```python
from build123d import *

# Parameters (mm, degrees)
BOARD_DEPTH        = 1.59936
CUT_EXTRUDE2_DEPTH = 2.59936
CUT_EXTRUDE3_DEPTH = 2.59936


with BuildPart() as part:
    # Sketch1 → Board (new body)
    with BuildSketch(Plane.XY):
        with BuildLine():
            Line((10, 12.987), (10, 24.35))
            ThreePointArc((10, 24.35), (10.089703362, 24.915270998), (10.35, 25.425))
            ThreePointArc((10.35, 25.425), (10.610296638, 25.934729002), (10.7, 26.5))
            Line((10.7, 26.5), (10.7, 27.5))
            ThreePointArc((10.7, 27.5), (10.610296638, 28.065270998), (10.35, 28.575))
            ThreePointArc((10.35, 28.575), (10.089703362, 29.084729002), (10, 29.65))
            Line((10, 29.65), (10, 41.1))
            ThreePointArc((10, 41.1), (10.089703362, 41.665270998), (10.35, 42.175))
            ThreePointArc((10.35, 42.175), (10.610296638, 42.684729002), (10.7, 43.25))
            Line((10.7, 43.25), (10.7, 44.25))
            ThreePointArc((10.7, 44.25), (10.610296638, 44.815270998), (10.35, 45.325))
            ThreePointArc((10.35, 45.325), (10.089703362, 45.834729002), (10, 46.4))
            Line((10, 46.4), (10, 57.01299))
            ThreePointArc((10, 57.01299), (10.185195521, 57.290150019), (10.51213, 57.22512))
            ThreePointArc((10.51213, 57.22512), (12.776257609, 57.223732391), (12.77487, 59.48786))
            ThreePointArc((12.77487, 59.48786), (12.709829188, 59.814802566), (12.987, 60))
            Line((12.987, 60), (37.01299, 60))
            ThreePointArc((37.01299, 60), (37.290150019, 59.814804479), (37.22512, 59.48787))
            ThreePointArc((37.22512, 59.48787), (37.223732391, 57.223742391), (39.48786, 57.22513))
            ThreePointArc((39.48786, 57.22513), (39.814807186, 57.290168899), (40, 57.01299))
            Line((40, 57.01299), (40, 12.987))
            ThreePointArc((40, 12.987), (39.814804479, 12.709839981), (39.48787, 12.77487))
            ThreePointArc((39.48787, 12.77487), (37.226515909, 12.773484091), (37.22513, 10.51213))
            ThreePointArc((37.22513, 10.51213), (37.290158106, 10.185190901), (37.01299, 10))
            Line((37.01299, 10), (12.987, 10))
            ThreePointArc((12.987, 10), (12.709839981, 10.185195521), (12.77487, 10.51213))
            ThreePointArc((12.77487, 10.51213), (12.773484091, 12.773484091), (10.51213, 12.77487))
            ThreePointArc((10.51213, 12.77487), (10.185195521, 12.709839981), (10, 12.987))
        make_face()
    extrude(amount=BOARD_DEPTH)

    # Sketch17 → Cut-Extrude2 (cut, through all)
    with BuildSketch(Plane.XY.offset(1.59936)):
        with BuildLine():
            Line((24.592, 58.964), (24.592, 57.764))
            ThreePointArc((24.592, 57.764), (24.292, 57.464), (23.992, 57.764))
            Line((23.992, 57.764), (23.992, 58.964))
            ThreePointArc((23.992, 58.964), (24.292, 59.264), (24.592, 58.964))
        make_face()
        with BuildLine():
            Line((24.592, 54.584), (24.592, 53.784))
            ThreePointArc((24.592, 53.784), (24.292, 53.484), (23.992, 53.784))
            Line((23.992, 53.784), (23.992, 54.584))
            ThreePointArc((23.992, 54.584), (24.292, 54.884), (24.592, 54.584))
        make_face()
        with BuildLine():
            Line((15.96453, 54.46518), (15.96453, 53.66518))
            ThreePointArc((15.96453, 53.66518), (15.66453, 53.36518), (15.36453, 53.66518))
            Line((15.36453, 53.66518), (15.36453, 54.46518))
            ThreePointArc((15.36453, 54.46518), (15.66453, 54.76518), (15.96453, 54.46518))
        make_face()
        with BuildLine():
            Line((15.956, 58.964), (15.956, 57.764))
            ThreePointArc((15.956, 57.764), (15.656, 57.464), (15.356, 57.764))
            Line((15.356, 57.764), (15.356, 58.964))
            ThreePointArc((15.356, 58.964), (15.656, 59.264), (15.956, 58.964))
        make_face()
    extrude(amount=-CUT_EXTRUDE2_DEPTH, mode=Mode.SUBTRACT)

    # Sketch18 → Cut-Extrude3 (cut, through all)
    with BuildSketch(Plane.XY.offset(1.59936)):
        with BuildLine():
            Line((37.015, 37.3), (41.715, 37.3))
            Line((41.715, 37.3), (41.715, 36.7))
            Line((41.715, 36.7), (37.015, 36.7))
            ThreePointArc((37.015, 36.7), (36.714999967, 37), (37.015, 37.3))
        make_face()
    extrude(amount=-CUT_EXTRUDE3_DEPTH, mode=Mode.SUBTRACT)


solid = part.part
```
Source: CAD feature listing. Evaluate the final solid. Frame: model axes, mm. A direction names the side the tool comes from. Give positions to 0.01 mm unless a question says otherwise; leave off trailing zeros. Loops run counter-clockwise (first coordinate to the right, second up) from the corner with the lowest first, then second, coordinate; pieces in that order, holes last. Notation, with made-up numbers: (13.5, -26.75) -> (34.5, -26.75) arc R21 cw to (34.5, 3.25) -> close; hole circle Ø8 at (84, 43.5). An arc over 180 degrees is marked (long way). Put each result on its own line as item: value. Start each with the question number.
1) Contact query for flat-ended pins moving along their axis: P1, Ø2, axis at x = 16, y = 37, coming from the -Z side; P2, Ø0.8, axis at x = 38.5, z = 0.5, coming from the -Y side; P3, Ø0.6, axis at y = 58.5, z = 1, coming from the +X side; P4, Ø0.8, axis at x = 38.5, z = 1, coming from the +Y side. Output: stop coordinate, or through.
2) Draft query along X for faces 5 (the face through (40, 47, 1)), 6 (the face through (24.592, 58, 1)), 7 (the face through (38, 37.3, 1)). Return one class per face: released by +X, released by -X, zero draft, split by the parting line, or undercut.
3) Reachability of faces 1 (the face through (40, 25, 1)), 2 (the face through (39, 36.7, 1)), 3 (the face through (10.7, 27, 1)), 4 (the face through (15.356, 58, 1)) from +Z, -Z, +X, -X, +Y, -Y: full face, straight path, thin tool, end or side. Return the list, or none.
4) Cut plane A-A (x = 38). Return loops of the section in (y, z), then the cut area to 3 significant figures.
5) Cut plane B-B (y = 28). Return loops of the section in (x, z), then the cut area to 3 significant figures.
6) Material intervals for probe 1 along X at (y, z) = (54, 1); probe 2 along X at (y, z) = (13, 1.1); probe 3 along X at (y, z) = (27.5, 0.8), sorted ascending.
Results are:
1. P1: stops at z = 0
1. P2: stops at y = 13.15
1. P3: stops at x = 36.82
1. P4: stops at y = 56.85
2. face 5: released by +X
2. face 6: undercut
2. face 7: zero draft
3. face 1: +Z, -Z, +X, +Y, -Y
3. face 2: +Z, -Z, +X
3. face 3: +Z, -Z, -X
3. face 4: +Z, -Z
4. outline: (13.2, 0) -> (36.7, 0) -> (36.7, 1.6) -> (13.2, 1.6) -> close; (37.3, 0) -> (56.8, 0) -> (56.8, 1.6) -> (37.3, 1.6) -> close
4. area: 68.8 mm2
5. outline: (10.63, 0) -> (40, 0) -> (40, 1.6) -> (10.63, 1.6) -> close
5. area: 47.0 mm2
6. probe 1: x = 10 to 15.36, 15.96 to 23.99, 24.59 to 40
6. probe 2: x = 10 to 10.8, 12.49 to 37.51, 39.2 to 40
6. probe 3: x = 10.7 to 40
